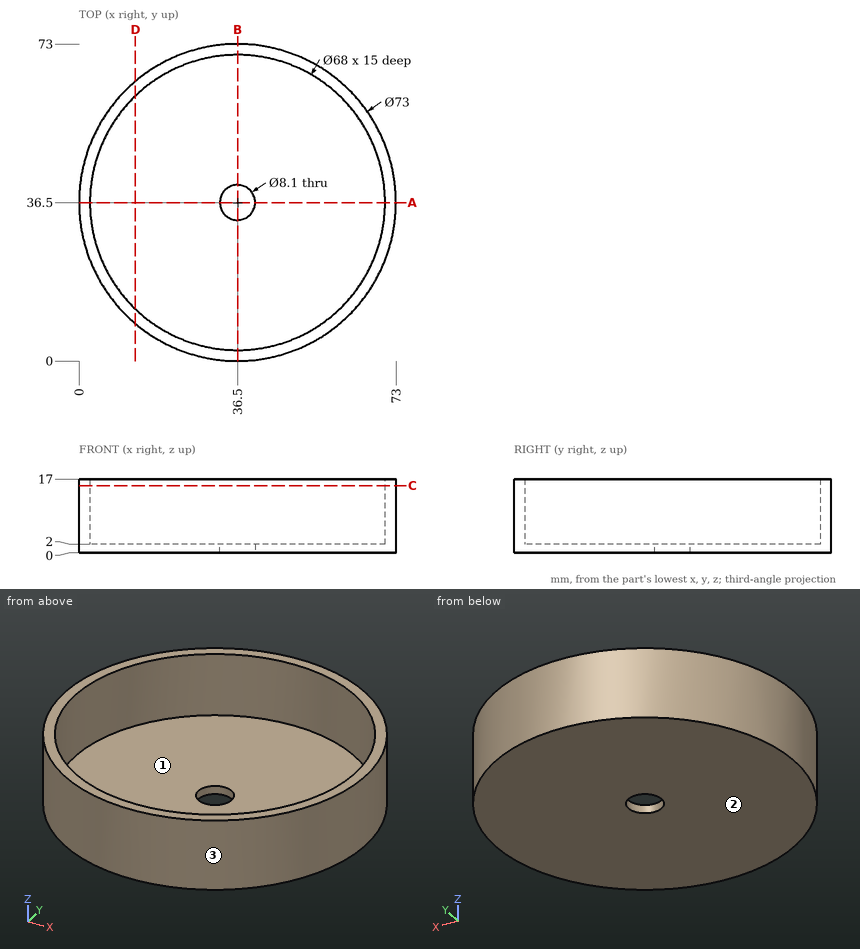
Geometry check sheet. Reference: drawing and pictorial views, mm from the part's lowest x, y, z. Give positions to 0.01 mm unless a question says otherwise; leave off trailing zeros. Write each loop counter-clockwise with the first axis right and the second up, starting at its lowest first coordinate (ties: lowest second). Pieces come first, ordered by that corner, then holes.
Item 1: Cross-section at D-D (x = 13). Enter the section's corners in (y, z).
Item 2: Gauge pin test, flat ends, axial feed: pin 1 (6 mm diameter, centred on x = 22, y = 22, fed in from -Z); pin 2 (1.5 mm diameter, centred on x = 55, z = 5, fed in from -Y); pin 3 (2 mm diameter, centred on y = 10.5, z = 5.5, fed in from -X); pin 4 (2 mm diameter, centred on x = 20, z = 7.5, fed in from +Y). Record the tip position at first contact, or that the pin passes through.
Item 3: Scan lines: L1, parallel to Y at x = 36.5, z = 9.5; L2, parallel to Y at x = 36.5, z = 0.55; L3, parallel to Z at x = 58, y = 11. Record each from-to range of solid material in increasing order.
Item 4: Cross-section at A-A (y = 36.5). Enter the section's corners in (x, z), and give its area (3 significant figures).
Item 5: Cross-section at C-C (z = 15.5). Enter the section's corners in (x, y), and give its area (3 significant figures).
Item 6: Draft check along X on the marked faces 1, 2 and 3. Enter one of: released by +X, released by -X, zero draft, split by the parting line, or undercut.
Report:
1. outline: (8.57, 0) - (64.43, 0) - (64.43, 17) - (61.07, 17) - (61.07, 2) - (11.93, 2) - (11.93, 17) - (8.57, 17) - close
2. pin 1: stops at z = 0
2. pin 2: stops at y = 4.61
2. pin 3: stops at x = 9.91
2. pin 4: stops at y = 69.55
3. L1: y = 0 to 2.5, 70.5 to 73
3. L2: y = 0 to 32.45, 40.55 to 73
3. L3: z = 0 to 2
4. outline: (0, 0) - (32.45, 0) - (32.45, 2) - (2.5, 2) - (2.5, 17) - (0, 17) - close; (40.55, 0) - (73, 0) - (73, 17) - (70.5, 17) - (70.5, 2) - (40.55, 2) - close
4. area: 205 mm2
5. outline: circle Ø73 at (36.5, 36.5); hole circle Ø68 at (36.5, 36.5)
5. area: 554 mm2
6. face 1: undercut
6. face 2: zero draft
6. face 3: split by the parting line
